Geometry check sheet. Reference: the model listing, model coordinates, mm. Give positions to 0.01 mm unless a question says otherwise; leave off trailing zeros. Order: outer loops, then holes, each group sorted by start corner. A loop starts at its lowest first (then second) coordinate and runs counter-clockwise, first axis right, second up. Notation, with made-up numbers: M -31.5,72.5 L -20.5,72.5 A18 ccw -20.5,102.5 Z; hole C 12.5,27.5 d10. An arc over 180 degrees is marked long. Put each result on its own line as item: value. Start each with the question number.
Q1. Section check D-D on y = 204. Record the cut outline in (x, z), then the cut area to 3 significant figures.
Q2. Mould release check, pull along X, two halves, no side actions. Record for faces 1 (the flat face through (-98.17, 233.18, -1.48)), 2 (the flat face through (118, -57, -3)), 3 (the cylindrical face through (100.291, -108.456, -1.479)): +X half, -X half, draft (parallel to the pull), parting line (faces both ways), or undercut.
Q3. Section check B-B on x = -46.5. Record the cut outline in (y, z).
Q4. Material ranges on L1, parallel to Y at x = 0, z = -0.85; L2, parallel to X at y = 4, z = -1.25; L3, parallel to X at y = 220, z = -0.45, recorded low to high.
Q5. Go/stop test with flat-tipped pins: pin 1 (14.5 mm diameter, centred on x = 0, y = -150, fed in from +Z); pin 2 (10 mm diameter, centred on x = -106.07, y = -106.07, fed in from -Z). Record where each tip stops, or that it passes through.
Q6. Section check C-C on z = -1.5. State how many separate pieces and enclosed holes the cut face has, then the cut area to 3 significant figures.
Q7. Section check A-A on y = 70.5. Record the cut outline in (x, z), then the cut area to 3 significant figures.
Autodesk Inventor part; units mm, degrees
ref_plane "YZ Plane" through (0, 0, 0) normal (1, 0, 0) x (0, 1, 0)
ref_plane "XZ Plane" through (0, 0, 0) normal (0, 1, 0) x (-1, 0, 0)
ref_plane "XY Plane" through (0, 0, 0) normal (0, 0, 1) x (1, 0, 0)
sketch "Sketch2" plane through (0, 0, 0) normal (0, 0, 1) x (1, 0, 0)
  line L0 (-193.6378, 193.6378) -> (0, 273.8452)
  line L1 (0, 273.8452) -> (193.6378, 193.6378)
  line L2 (193.6378, 193.6378) -> (273.8452, 0)
  line L3 (273.8452, 0) -> (193.6378, -193.6378)
  line L4 (193.6378, -193.6378) -> (0, -273.8452)
  line L5 (0, -273.8452) -> (-193.6378, -193.6378)
  line L6 (-193.6378, -193.6378) -> (-273.8452, 0)
  line L7 (-273.8452, 0) -> (-193.6378, 193.6378)
  circle A0 centre (0, 0) radius 130
  dimension "d23" = 506
  dimension "d26" = 260
extrude "Plate1" add sketch "Sketch2" against normal blind 3
sketch "Sketch4" plane through (0, 0, 0) normal (0, 0, 1) x (1, 0, 0)
  circle A0 centre (0, 150) radius 6.25
  circle A1 centre (0, 0) radius 130
  dimension "d16" = 12.5
  dimension "d17" = 150
extrude "Extrusion1" cut sketch "Sketch4" against normal up to surface (3 mm away) contours A0
pattern_circular "Circular Pattern1" count 8 over 360 about axis through (0, 0, -10) along (0, 0, 1) of "Extrusion1"
equation "\"d23\" = Барабан_габарит_по_кассетам"
equation "\"d26\" = Вал_ось_диаметр_НОС"
equation "\"d15\" = Thickness"
equation "\"BendRadius\" = Thickness"
equation "\"BendReliefWidth\" = Thickness"
equation "\"BendReliefDepth\" = 0.5 * Thickness"
equation "\"CornerReliefSize\" = 4 * Thickness"
equation "\"MinimumRemnant\" = 2 * Thickness"
equation "\"TransitionRadius\" = BendRadius"
equation "\"JacobiRadiusSize\" = BendRadius"
equation "\"GapSize\" = Thickness"
properties part number "ДМС 101 Барабан торец"
Results found:
1. outline: M -168.62,-3 L 168.62,-3 L 168.62,0 L -168.62,0 Z
1. area: 1,010 mm^2
2. face 1: -X half
2. face 2: draft
2. face 3: undercut
3. outline: M -254.58,-3 L -121.4,-3 L -121.4,0 L -254.58,0 Z; M 121.4,-3 L 254.58,-3 L 254.58,0 L 121.4,0 Z
4. L1: y = -273.85 to -156.25, -143.75 to -130, 130 to 143.75, 156.25 to 273.85
4. L2: x = -272.19 to -154.8, -145.2 to -129.94, 129.94 to 145.2, 154.8 to 272.19
4. L3: x = -129.99 to 129.99
5. pin 1: stops at z = 0
5. pin 2: passes through
6. separate pieces: 1
6. enclosed holes: 9
6. area: 158,000 mm^2
7. outline: M -244.64,-3 L -109.22,-3 L -109.22,0 L -244.64,0 Z; M 109.22,-3 L 244.64,-3 L 244.64,0 L 109.22,0 Z
7. area: 813 mm^2
